Part model, mm, in its own coordinate system. A direction names the side the tool comes from. Coordinates: 2 decimals unless noted, no trailing zeros. Use a Markdown table: item, result. Add a question column.
Q1. Mould opens along Y. For faces 1 (the cylindrical face through (-403.227, -41.415, -0.089)), 2 (the flat face through (-6, -63.5, 0)), 3 (the flat face through (-6, 1, 6.35)) say: released by +Y, released by -Y, zero draft, split by the parting line, or undercut.
Q2. Pin check, flat tip, straight feed: pin 1 Ø3.5 at (y, z) = (44, -4.5) entering from -X. Stop position of the tip, or through.
Q3. Tool access for faces 4 (the flat face through (-375, 45, -3.175)), 5 (the flat face through (-415.925, -56, 0)): list every direction of +Z, -Z, +X, -X, +Y, -Y with a clear straight run to the whole face (end or side of a thin tool).
Q4. Wall check: L1, parallel to X at y = 56.5, z = 1.25 (3 decimals); L2, parallel to X at y = 58, z = -5.5 (3 decimals); L3, parallel to Y at x = -381, z = 3.5. Give the ranges that are in metal, low to high. Write a range as from..to.
from build123d import *

# Parameters (mm, degrees)
SKETCH1_W                         = 831.85
SKETCH1_H                         = 127
BOSS_EXTRUDE1_DEPTH               = 6.35
F_10_CLEARANCE_HOLE1_D            = 5.1054
TAPPED_HOLE_FOR_10_32_HELICOIL1_D = 5.1054
LPATTERN1_COUNT                   = 5
LPATTERN1_PITCH                   = 171.45
CUT_EXTRUDE1_DEPTH                = 421.936035075
CUT_EXTRUDE3_REACH                = 422.936
CUT_EXTRUDE4_DEPTH                = 3.175


with BuildPart() as part:
    # Sketch1 → Boss-Extrude1 (new, symmetric)
    with BuildSketch(Plane.XY):
        Rectangle(SKETCH1_W, SKETCH1_H)
    extrude(amount=BOSS_EXTRUDE1_DEPTH, both=True)

    # #10 Clearance Hole1 (through all)
    with Locations(Plane(origin=(0, 0, -6.35), x_dir=(-1, 0, 0), z_dir=(0, 0, -1))):
        with Locations((-409.575, 57.15), (-409.575, -57.15)):
            f_10_clearance_hole1 = Hole(F_10_CLEARANCE_HOLE1_D / 2)

    # Tapped Hole for #10-32 Helicoil1 (through all)
    with Locations(Plane(origin=(0, 0, -6.35), x_dir=(-1, 0, 0), z_dir=(0, 0, -1))):
        with Locations((-381, 10.38225), (-304.8, -10.38225)):
            tapped_hole_for_10_32_helicoil1 = Hole(TAPPED_HOLE_FOR_10_32_HELICOIL1_D / 2)

    # LPattern1: Tapped Hole for #10-32 Helicoil1 ×5, 1 skipped
    with Locations(*[(-i * LPATTERN1_PITCH, 0, 0) for i in range(1, LPATTERN1_COUNT) if i not in (2,)]):
        add(tapped_hole_for_10_32_helicoil1, mode=Mode.SUBTRACT)

    # Sketch9 → Cut-Extrude1 (cut, through all)
    with BuildSketch(Plane(origin=(0, 0, -6.35), x_dir=(-1, 0, 0), z_dir=(0, 0, -1))):
        with BuildLine():
            Line((-422.275, 47.625), (-409.575, 47.625))
            ThreePointArc((-409.575, 47.625), (-403.225, 41.275), (-409.575, 34.925))
            Line((-409.575, 34.925), (-422.275, 34.925))
            ThreePointArc((-422.275, 34.925), (-428.625, 41.275), (-422.275, 47.625))
        make_face()
        with BuildLine():
            Line((-422.275, -47.625), (-409.575, -47.625))
            ThreePointArc((-409.575, -47.625), (-403.225, -41.275), (-409.575, -34.925))
            Line((-409.575, -34.925), (-422.275, -34.925))
            ThreePointArc((-422.275, -34.925), (-428.625, -41.275), (-422.275, -47.625))
        make_face()
    cut_extrude1 = extrude(amount=-CUT_EXTRUDE1_DEPTH, mode=Mode.SUBTRACT)

    # Mirror1: #10 Clearance Hole1, Cut-Extrude1 across plane
    add(f_10_clearance_hole1.mirror(Plane(origin=(0, 0, 0), x_dir=(0, 0, 1), z_dir=(1, 0, 0))), mode=Mode.SUBTRACT)
    add(cut_extrude1.mirror(Plane(origin=(0, 0, 0), x_dir=(0, 0, 1), z_dir=(1, 0, 0))), mode=Mode.SUBTRACT)

    # Sketch13 → Cut-Extrude3 (cut, up to next)
    with BuildSketch(Plane.XY.offset(6.35), mode=Mode.PRIVATE) as cut_extrude3_sk1:
        with BuildLine():
            Line((-372.618, 60.2615), (-366.268, 60.2615))
            ThreePointArc((-366.268, 60.2615), (-364.6805, 58.674), (-366.268, 57.0865))
            Line((-366.268, 57.0865), (-372.618, 57.0865))
            ThreePointArc((-372.618, 57.0865), (-374.2055, 58.674), (-372.618, 60.2615))
        make_face()
    cut_extrude3_tool1 = extrude(cut_extrude3_sk1.sketch, amount=-CUT_EXTRUDE3_REACH, mode=Mode.PRIVATE) & part.part
    # Sketch13 → Cut-Extrude3 (cut, up to next)
    with BuildSketch(Plane.XY.offset(6.35), mode=Mode.PRIVATE) as cut_extrude3_sk2:
        with BuildLine():
            Line((-383.032, 38.1635), (-376.682, 38.1635))
            ThreePointArc((-376.682, 38.1635), (-375.0945, 36.576), (-376.682, 34.9885))
            Line((-376.682, 34.9885), (-383.032, 34.9885))
            ThreePointArc((-383.032, 34.9885), (-384.6195, 36.576), (-383.032, 38.1635))
        make_face()
    cut_extrude3_tool2 = extrude(cut_extrude3_sk2.sketch, amount=-CUT_EXTRUDE3_REACH, mode=Mode.PRIVATE) & part.part
    # Sketch13 → Cut-Extrude3 (cut, up to next)
    with BuildSketch(Plane.XY.offset(6.35), mode=Mode.PRIVATE) as cut_extrude3_sk3:
        with BuildLine():
            Line((302.768, 60.2615), (309.118, 60.2615))
            ThreePointArc((309.118, 60.2615), (310.7055, 58.674), (309.118, 57.0865))
            Line((309.118, 57.0865), (302.768, 57.0865))
            ThreePointArc((302.768, 57.0865), (301.1805, 58.674), (302.768, 60.2615))
        make_face()
    cut_extrude3_tool3 = extrude(cut_extrude3_sk3.sketch, amount=-CUT_EXTRUDE3_REACH, mode=Mode.PRIVATE) & part.part
    # Sketch13 → Cut-Extrude3 (cut, up to next)
    with BuildSketch(Plane.XY.offset(6.35), mode=Mode.PRIVATE) as cut_extrude3_sk4:
        with BuildLine():
            Line((313.182, 38.1635), (319.532, 38.1635))
            ThreePointArc((319.532, 38.1635), (321.1195, 36.576), (319.532, 34.9885))
            Line((319.532, 34.9885), (313.182, 34.9885))
            ThreePointArc((313.182, 34.9885), (311.5945, 36.576), (313.182, 38.1635))
        make_face()
    cut_extrude3_tool4 = extrude(cut_extrude3_sk4.sketch, amount=-CUT_EXTRUDE3_REACH, mode=Mode.PRIVATE) & part.part
    add(cut_extrude3_tool1.solids().sort_by_distance((-369.443, 58.674, 6.35))[0], mode=Mode.SUBTRACT)
    add(cut_extrude3_tool2.solids().sort_by_distance((-379.857, 36.576, 6.35))[0], mode=Mode.SUBTRACT)
    add(cut_extrude3_tool3.solids().sort_by_distance((305.943, 58.674, 6.35))[0], mode=Mode.SUBTRACT)
    add(cut_extrude3_tool4.solids().sort_by_distance((316.357, 36.576, 6.35))[0], mode=Mode.SUBTRACT)

    # Sketch14 → Cut-Extrude4 (cut)
    with BuildSketch(Plane(origin=(0, 0, -6.35), x_dir=(-1, 0, 0), z_dir=(0, 0, -1))):
        with BuildLine():
            Line((-330.2, 63.5), (-292.1, 63.5))
            Line((-292.1, 63.5), (-292.1, 31.75))
            ThreePointArc((-292.1, 31.75), (-293.959871939, 27.259871939), (-298.45, 25.4))
            Line((-298.45, 25.4), (-323.85, 25.4))
            ThreePointArc((-323.85, 25.4), (-328.340128061, 27.259871939), (-330.2, 31.75))
            Line((-330.2, 31.75), (-330.2, 63.5))
        make_face()
        with BuildLine():
            Line((355.6, 63.5), (393.7, 63.5))
            Line((393.7, 63.5), (393.7, 31.75))
            ThreePointArc((393.7, 31.75), (391.840128061, 27.259871939), (387.35, 25.4))
            Line((387.35, 25.4), (361.95, 25.4))
            ThreePointArc((361.95, 25.4), (357.459871939, 27.259871939), (355.6, 31.75))
            Line((355.6, 31.75), (355.6, 63.5))
        make_face()
    extrude(amount=-CUT_EXTRUDE4_DEPTH, mode=Mode.SUBTRACT)


solid = part.part
Recorded:
| question | item | result |
|---|---|---|
| 1 | face 1 | undercut |
| 1 | face 2 | released by -Y |
| 1 | face 3 | zero draft |
| 2 | pin 1 | x = -405.07 |
| 3 | face 4 | -Z, +Y |
| 3 | face 5 | +Z, -Z, -X, +Y, -Y |
| 4 | L1 | -415.925..-412.044, -407.106..407.106, 412.044..415.925 |
| 4 | L2 | -415.925..-411.982, -407.168..-393.7, -355.6..292.1, 330.2..407.168, 411.982..415.925 |
| 4 | L3 | -63.5..-12.93, -7.83..34.99, 38.16..63.5 |
